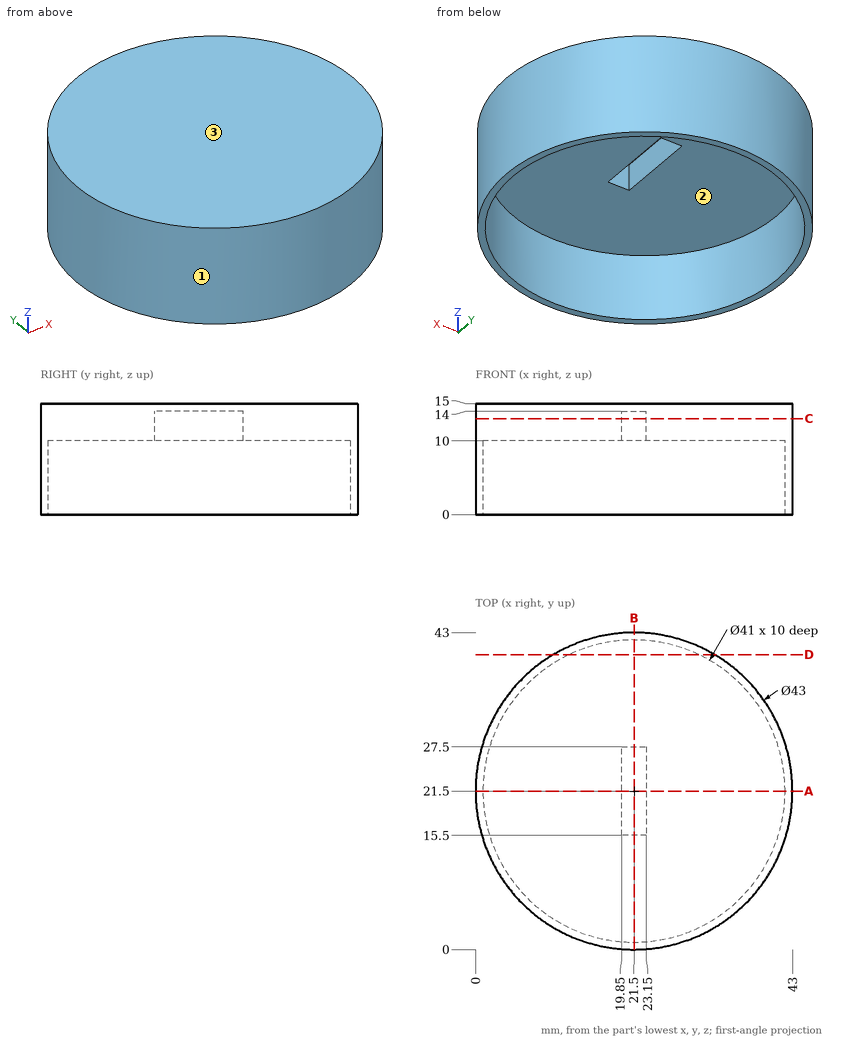
Drawing for the job (mm, zero at the part's lowest x, y, z). Round coordinates to 2 decimals unless told otherwise and drop trailing zeros. Write each loop counter-clockwise with the first axis right and the second up, starting at its lowest first coordinate (ties: lowest second). Pieces come first, ordered by that corner, then holes. Notation, with made-up numbers: (33.25, 25.5) - (39.25, 25.5) arc R21 cw to (39.25, 57.5) - close; hole circle Ø8 at (-24, 28.5). An arc over 180 degrees is marked (long way). Return JSON: item names as keys, results as strings. Group by question number.
Item 1: Band-saw the part on B-B on x = 21.5. List the corners of the cut face in (y, z).
Item 2: Mould opens along Y. For the marked faces 1, 2 and 3 say: +Y half, -Y half, draft (parallel to the pull), parting line (faces both ways), or undercut.
Item 3: Flat gauge pins, fed straight in: pin 1 Ø12.5 at (x, y) = (30.5, 15.5) entering from -Z; pin 2 Ø1 at (y, z) = (30, 5) entering from +X; pin 3 Ø2 at (x, z) = (20, 6) entering from +Y. Where does each tip first touch, or does it go through?
Item 4: Band-saw the part on A-A on y = 21.5. List the corners of the cut face in (x, z).
Item 5: Band-saw the part on C-C on z = 13. List the corners of the cut face in (x, y).
Item 6: Band-saw the part on D-D on y = 40. List the corners of the cut face in (x, z), plus the area to 3 significant figures.
Item 7: Probe probe 1 along Y at (x, z) = (21.5, 7.5); probe 2 along Y at (x, z) = (21.5, 12.5); probe 3 along Z at (x, y) = (29, 18.5). List the from-to ranges inside material, lowest first.
Resolved:
{
 "1": {"outline": "(0, 0) - (1, 0) - (1, 10) - (15.5, 10) - (15.5, 14) - (27.5, 14) - (27.5, 10) - (42, 10) - (42, 0) - (43, 0) - (43, 15) - (0, 15) - close"},
 "2": {"face 1": "parting line", "face 2": "undercut", "face 3": "draft"},
 "3": {"pin 1": "stops at z = 10", "pin 2": "stops at x = 41.46", "pin 3": "stops at y = 42.99"},
 "4": {"outline": "(0, 0) - (1, 0) - (1, 10) - (19.85, 10) - (19.85, 14) - (23.15, 14) - (23.15, 10) - (42, 10) - (42, 0) - (43, 0) - (43, 15) - (0, 15) - close"},
 "5": {"outline": "circle Ø43 at (21.5, 21.5); hole (19.85, 15.5) - (23.15, 15.5) - (23.15, 27.5) - (19.85, 27.5) - close"},
 "6": {"outline": "(10.55, 0) - (12.67, 0) - (12.67, 10) - (30.33, 10) - (30.33, 0) - (32.45, 0) - (32.45, 15) - (10.55, 15) - close", "area": "152 mm²"},
 "7": {"probe 1": "y = 0 to 1, 42 to 43", "probe 2": "y = 0 to 15.5, 27.5 to 43", "probe 3": "z = 10 to 15"}
}
